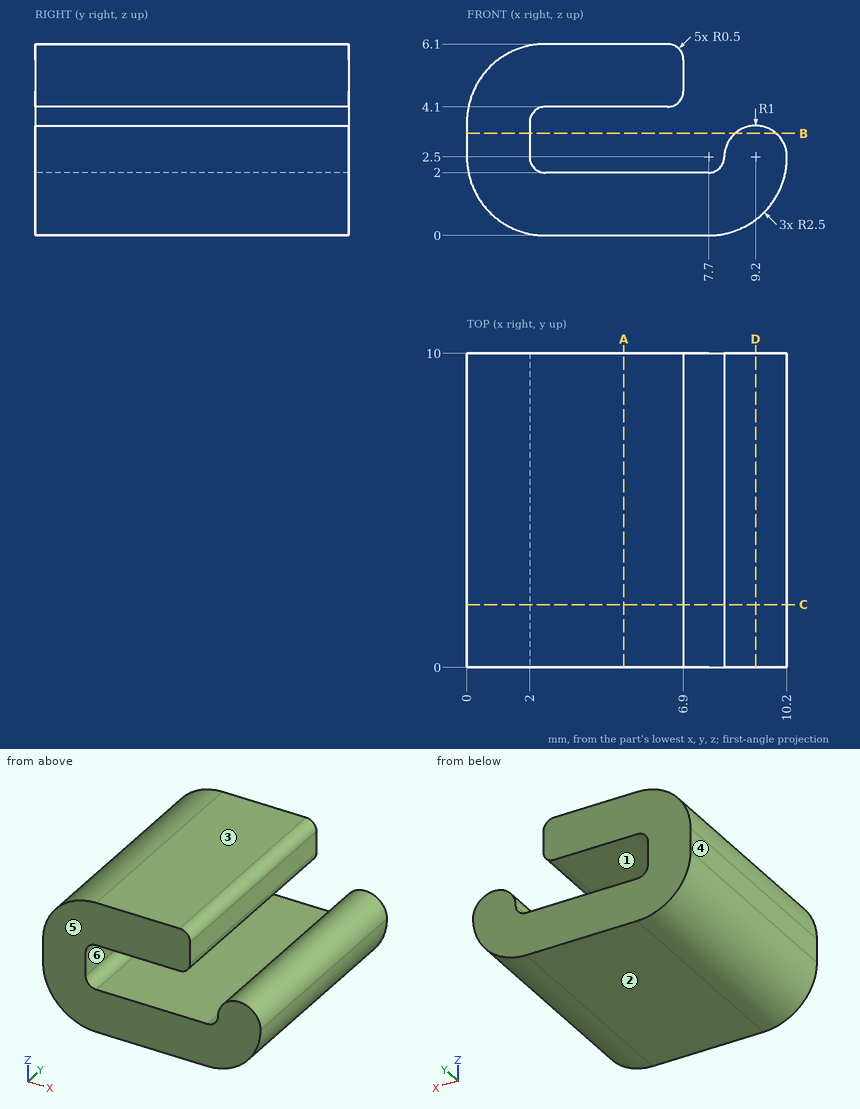
Could you check a few things on this drawing? It's one solid part, dimensions in mm from its lowest x, y, z. A direction names the side the tool comes from. Give positions to 0.01 mm unless a question says otherwise; leave off trailing zeros. Loops run counter-clockwise (first coordinate to the right, second up) from the corner with the lowest first, then second, coordinate; pieces in that order, holes last. Notation, with made-up numbers: M 62,63 L 82,63 A23 ccw 82,88 Z; hole C 69.25,58.25 d3. An arc over 180 degrees is marked long. One line per question, with ' | ' between items. Start each with the question number.
Q1. If we section it at A-A (x = 5): Please give me the cut outline in (y, z).
Q2. For the marked faces 5 and 6, which set-ups out of +Z, -Z, +X, -X, +Y, -Y let a thin tool reach every point of the face, with its end or its side?
Q3. For pin 1 Ø3 at (y, z) = (2.5, 1) entering from +X; pin 2 Ø0.5 at (y, z) = (3, 5) entering from +X, each with a flat end and sliding along its axis, tell me the tip position at first contact or that it passes through.
Q4. If I drill on line 1 (Z direction, x = 6, y = 1.25); line 2 (X direction, y = 1.75, z = 3.25); line 3 (Z direction, x = 1.25, y = 0.5), over which ranges is the centre line in solid material (lowest first)? Write a range as from..to.
Q5. If we section it at C-C (y = 2): Please give me the cut outline in (x, z), plus the area to 3 significant figures.
Q6. If we section it at B-B (z = 3.25): Please give me the cut outline in (x, y).
Q7. If we section it at D-D (x = 9.2): Please give me the cut outline in (y, z).
Q8. If we mould it in two halves opening along Z, with no side actions, what happens to the marked faces 1, 2, 3 and 4? For each: +Z half, -Z half, draft (parallel to the pull), parting line (faces both ways), or undercut.
Computed:
1) outline: M 0,0 L 10,0 L 10,2 L 0,2 Z; M 0,4.1 L 10,4.1 L 10,6.1 L 0,6.1 Z
2) face 5: +Z, -Z, +X, -X, -Y | face 6: +Y, -Y
3) pin 1: stops at x = 10.2 | pin 2: stops at x = 6.9
4) line 1: z = 0..2, 4.1..6.1 | line 2: x = 0..2, 8.54..9.86 | line 3: z = 0.33..5.77
5) outline: M 0,2.5 A2.5 ccw 2.5,0 L 7.7,0 A2.5 ccw 10.2,2.5 A1 ccw 8.2,2.5 A0.5 cw 7.7,2 L 2.5,2 A0.5 cw 2,2.5 L 2,3.6 A0.5 cw 2.5,4.1 L 6.4,4.1 A0.5 ccw 6.9,4.6 L 6.9,5.6 A0.5 ccw 6.4,6.1 L 2.5,6.1 A2.5 ccw 0,3.6 Z | area: 37.0 mm²
6) outline: M 0,0 L 2,0 L 2,10 L 0,10 Z; M 8.54,0 L 9.86,0 L 9.86,10 L 8.54,10 Z
7) outline: M 0,0.5 L 10,0.5 L 10,3.5 L 0,3.5 Z
8) face 1: undercut | face 2: -Z half | face 3: +Z half | face 4: draft
